Part model, mm, in its own coordinate system. Face numbers are marked on the shaded views. A direction names the side the tool comes from. Coordinates: 2 decimals unless noted, no trailing zeros. Order: outer loops, then holes, each group sorted by start corner. A loop starts at its lowest first (then second) coordinate and runs counter-clockwise, first axis right, second up.
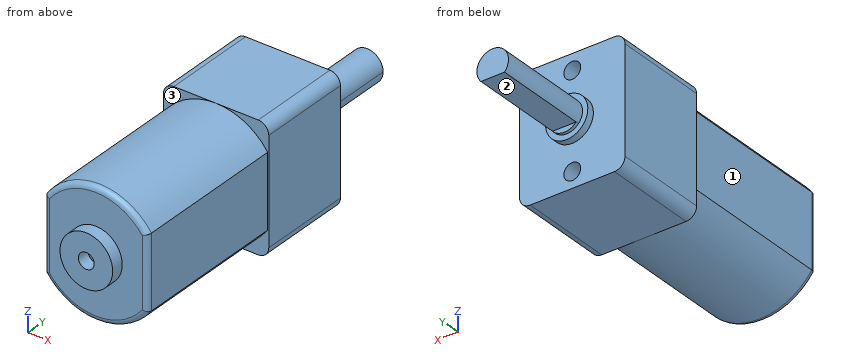
```python
from build123d import *

# Parameters (mm, degrees)
SKETCH_1_W      = 10
SKETCH_1_H      = 12
SKETCH_1_R      = 2
SKETCH_1_R_2    = 0.8
EXTRUDE_1_DEPTH = 9
SKETCH_1_3_R    = 2
SKETCH_1_3_R_2  = 1.5
EXTRUDE_3_DEPTH = 9.7
EXTRUDE_4_DEPTH = 19
SKETCH_1_5_R    = 1.5
EXTRUDE_5_DEPTH = 10
EXTRUDE_6_DEPTH = 15.1
SKETCH_4_R      = 2.5
SKETCH_4_R_2    = 0.75
EXTRUDE_7_DEPTH = 1.2
FILLET_1_R      = 1
FILLET_2_R      = 0.5


with BuildPart() as part:
    # 草图1 → 凸台-拉伸1 (new body)
    with BuildSketch(Plane(origin=(0, 0, 0), x_dir=(1, 0, 0), z_dir=(0, 1, 0))):
        Rectangle(SKETCH_1_W, SKETCH_1_H)
        with Locations(Location((0, 0, 0), (0, 0, 270))):
            Circle(SKETCH_1_R, mode=Mode.SUBTRACT)
        with Locations(Location((0, -4.5, 0), (0, 0, 270))):
            Circle(SKETCH_1_R_2, mode=Mode.SUBTRACT)
        with Locations(Location((0, 4.5, 0), (0, 0, 270))):
            Circle(SKETCH_1_R_2, mode=Mode.SUBTRACT)
    extrude(amount=EXTRUDE_1_DEPTH)

    # 草图1<3> → 凸台-拉伸3 (add)
    with BuildSketch(Plane(origin=(0, 0, 0), x_dir=(1, 0, 0), z_dir=(0, 1, 0))):
        with Locations(Location((0, 0, 0), (0, 0, 270))):
            Circle(SKETCH_1_3_R)
        with Locations(Location((0, 0, 0), (0, 0, 270))):
            Circle(SKETCH_1_3_R_2, mode=Mode.SUBTRACT)
    extrude(amount=EXTRUDE_3_DEPTH)

    # 草图1<4> → 凸台-拉伸4 (add)
    with BuildSketch(Plane(origin=(0, 0, 0), x_dir=(1, 0, 0), z_dir=(0, 1, 0))):
        with BuildLine():
            Line((1.118033989, 1), (-1.118033989, 1))
            ThreePointArc((-1.118033989, 1), (-0.535233135, -1.401258538), (1.5, 0))
            ThreePointArc((1.5, 0), (1.401258538, 0.535233135), (1.118033989, 1))
        make_face()
    extrude(amount=EXTRUDE_4_DEPTH)

    # 草图1<5> → 凸台-拉伸5 (add)
    with BuildSketch(Plane(origin=(0, 0, 0), x_dir=(1, 0, 0), z_dir=(0, 1, 0))):
        with Locations(Location((0, 0, 0), (0, 0, 138.189685104))):
            Circle(SKETCH_1_5_R)
    extrude(amount=EXTRUDE_5_DEPTH)

    # 草图3 → 凸台-拉伸6 (add)
    with BuildSketch(Plane.XZ):
        with BuildLine():
            Line((4.9, -3.462657939), (4.9, 3.462657939))
            ThreePointArc((4.9, 3.462657939), (0, 6), (-4.9, 3.462657939))
            Line((-4.9, 3.462657939), (-4.9, -3.462657939))
            ThreePointArc((-4.9, -3.462657939), (0, -6), (4.9, -3.462657939))
        make_face()
    extrude(amount=EXTRUDE_6_DEPTH)

    # 草图4 → 凸台-拉伸7 (add)
    with BuildSketch(Plane.XZ.offset(15.1)):
        with Locations(Location((0, 0, 0), (0, 0, 270))):
            Circle(SKETCH_4_R)
        with Locations(Location((0, 0, 0), (0, 0, 270))):
            Circle(SKETCH_4_R_2, mode=Mode.SUBTRACT)
    extrude(amount=EXTRUDE_7_DEPTH)

    # 圆角1
    fillet_1_edges = [part.edges().sort_by_distance(p)[0] for p in [
        (5, 4.5, 6),
        (-5, 4.5, 6),
        (-5, 4.5, -6),
        (5, 4.5, -6),
    ]]
    fillet(fillet_1_edges, radius=FILLET_1_R)

    # 圆角2
    fillet_2_edges = [part.edges().sort_by_distance(p)[0] for p in [
        (0, -15.1, 6),
        (-4.9, -15.1, 0),
        (0, -15.1, -6),
        (4.9, -15.1, 0),
    ]]
    fillet(fillet_2_edges, radius=FILLET_2_R)


solid = part.part
```
(1) Slice it at C-C, the plane y = 11. Give the cut face in (x, z), then the cut area to 3 significant figures.
(2) Drop flat-ended pins along their axis: pin 1 (3.5 mm diameter, centred on y = -5.5, z = 0.5, fed in from +X); pin 2 (1.8 mm diameter, centred on x = 0, y = 16, fed in from -Z); pin 3 (2 mm diameter, centred on y = -4.5, z = -1, fed in from -X). Give the stop position or say it passes through.
(3) Slice it at A-A, the plane y = 5. Give the cut face in (x, z).
(4) Slice it at B-B, the plane y = -4. Give the cut face in (x, z).
(5) Tool access for the marked faces 1, 2 and 3: list every direction of +Z, -Z, +X, -X, +Y, -Y with a clear straight run to the whole face (end or side of a thin tool).
(6) Probe line 1 (X direction, y = 2.5, z = -4.5); line 2 (Z direction, x = -0.5, y = 8.5); line 3 (X direction, y = -15.85, z = 0). List the from-to ranges inside material, lowest first.
Here are the results:
1. outline: (-1.12, -1) - (1.12, -1) arc R1.5 ccw (long way) to start
1. area: 6.29 mm2
2. pin 1: stops at x = 4.9
2. pin 2: stops at z = -1
2. pin 3: stops at x = -4.9
3. outline: (-5, -5) arc R1 ccw to (-4, -6) - (4, -6) arc R1 ccw to (5, -5) - (5, 5) arc R1 ccw to (4, 6) - (-4, 6) arc R1 ccw to (-5, 5) - close; hole circle Ø1.6 at (0, -4.5); hole circle Ø1.6 at (0, 4.5)
4. outline: (-4.9, -3.46) arc R6 ccw to (4.9, -3.46) - (4.9, 3.46) arc R6 ccw to (-4.9, 3.46) - close
5. face 1: +Z, -Z, -X, -Y
5. face 2: -Z, +X, -X, +Y
5. face 3: -X, -Y
6. line 1: x = -5 to -0.8, 0.8 to 5
6. line 2: z = -6 to -5.12, -3.88 to 3.88, 5.12 to 6
6. line 3: x = -2.5 to -0.75, 0.75 to 2.5
